Verification items for the finished model (mm, model axes). A direction names the side the tool comes from. Round coordinates to 2 decimals unless told otherwise and drop trailing zeros. Order: outer loops, then holes, each group sorted by start corner. A loop starts at its lowest first (then second) coordinate and runs counter-clockwise, first axis right, second up. Notation, with made-up numbers: M 40,52 L 83,52 A19 ccw 83,84 Z; hole C -28,9.5 d5. An arc over 180 degrees is marked long. Return JSON: item names as keys, results as strings. Group by question number.
from build123d import *

# Parameters (mm, degrees)
F2_DEPTH = 35.179
F1_R     = 16.51
F3_DEPTH = 30.48
F5_DEPTH = 2


with BuildPart() as f2:
    # F0 (on Front) → F2 (new body, symmetric)
    with BuildSketch(Plane.XZ):
        Polygon((-35.56, 14.3), (-24.13, 0), (24.13, 0), (35.56, 14.3), (35.56, 27), (-35.56, 27), align=None)
    extrude(amount=F2_DEPTH, both=True)

    # F1 (on Front) → F3 (join, symmetric)
    with BuildSketch(Plane.XZ):
        with Locations((17.78, 19.05)):
            Circle(F1_R)
        with Locations((-17.78, 19.05)):
            Circle(F1_R)
    extrude(amount=F3_DEPTH, both=True)

    # F4 (on face) → F5 (cut)
    with BuildSketch(Plane(origin=(0, 0, 0), x_dir=(1, 0, 0), z_dir=(0, 0, -1))):
        with BuildLine():
            ThreePointArc((6.13, 23.179), (4.63, 24.679), (3.13, 23.179))
            Line((3.13, 23.179), (3.13, 20.179))
            ThreePointArc((3.13, 20.179), (4.63, 18.679), (6.13, 20.179))
            Line((6.13, 20.179), (6.13, 23.179))
        make_face()
        with BuildLine():
            ThreePointArc((-7.13, -22.179), (-8.63, -23.679), (-7.13, -25.179))
            Line((-7.13, -25.179), (-4.13, -25.179))
            ThreePointArc((-4.13, -25.179), (-2.63, -23.679), (-4.13, -22.179))
            Line((-4.13, -22.179), (-7.13, -22.179))
        make_face()
    extrude(amount=-F5_DEPTH, mode=Mode.SUBTRACT)


solid = f2.part
1. Draft check along Y on faces 4 (the face through (4.6, -18.68, 0.99)), 5 (the face through (-35.56, 0, 21)), 6 (the face through (0, 35.179, 14)), 7 (the face through (18, -30.48, 30)). Enter one of: +Y half, -Y half, draft (parallel to the pull), parting line (faces both ways), or undercut.
2. Cross-section at A-A (y = -29.5). Enter the section's corners in (x, z).
3. Go/stop test with flat-tipped pins: pin 1 (5 mm diameter, centred on x = 19, z = 30, fed in from +Y); pin 2 (8 mm diameter, centred on x = -25.5, y = 8.5, fed in from +Z); pin 3 (0.9 mm diameter, centred on x = 5, y = -21, fed in from -Z). Record where each tip stops, or that it passes through.
4. Cross-section at C-C (x = 28.5). Enter the section's corners in (y, z), plus the area to 3 significant figures.
5. Cross-section at D-D (z = 8.5). Enter the section's corners in (x, y).
6. Access from +Z, -Z, +X, -X, +Y, -Y to the whole of each face (thin tool, end or side, straight path). Record for faces 1 (the face through (6.13, -22, 1)), 2 (the face through (-18, -30.48, 30)), 3 (the face through (18, 30.48, 30)).
7. Thickness scan on line 1 along Y through (x, z) = (23, 29); line 2 along Z through (x, y) = (-17, 13.5); line 3 along X through (y, z) = (-16.5, 33.5). Record the ranges inside material, lowest first. Write a range as from..to.
8. Cross-section at B-B (x = 17). Enter the section's corners in (y, z), plus the area to 3 significant figures.
Computed:
{
 "1": {"face 4": "undercut", "face 5": "draft", "face 6": "+Y half", "face 7": "-Y half"},
 "2": {"outline": "M -35.56,14.3 L -24.13,0 L 24.13,0 L 35.56,14.3 L 35.56,27 L 32.25,27 A16.51 ccw 3.31,27 L -3.31,27 A16.51 ccw -32.25,27 L -35.56,27 Z"},
 "3": {"pin 1": "stops at y = 30.48", "pin 2": "stops at z = 35.14", "pin 3": "stops at z = 2"},
 "4": {"outline": "M -35.18,5.47 L 35.18,5.47 L 35.18,27 L 30.48,27 L 30.48,31.61 L -30.48,31.61 L -30.48,27 L -35.18,27 Z", "area": "1,800 mm²"},
 "5": {"outline": "M -30.92,-35.18 L 30.92,-35.18 L 30.92,35.18 L -30.92,35.18 Z"},
 "6": {"face 1": "-Z", "face 2": "+Z, +X, -X, -Y", "face 3": "+Z, +X, -X, +Y"},
 "7": {"line 1": "y = -30.48..30.48", "line 2": "z = 0..35.54", "line 3": "x = -25.77..-9.79, 9.79..25.77"},
 "8": {"outline": "M -35.18,0 L 35.18,0 L 35.18,27 L 30.48,27 L 30.48,35.54 L -30.48,35.54 L -30.48,27 L -35.18,27 Z", "area": "2,420 mm²"}
}
